from build123d import *

# Parameters (mm, degrees)
F0_W     = 20
F0_H     = 20
F0_W_2   = 9
F0_H_2   = 9
F1_DEPTH = 2
F2_W     = 20
F2_H     = 20
F3_DEPTH = 5.3
F4_R     = 5.25
F5_DEPTH = 10


with BuildPart() as f1:
    # F0 (on Top) → F1 (new body)
    with BuildSketch(Plane.XY):
        Rectangle(F0_W, F0_H)
        Rectangle(F0_W_2, F0_H_2, mode=Mode.SUBTRACT)
    extrude(amount=F1_DEPTH)

    # F2 (on face) → F3 (join)
    with BuildSketch(Plane.XY.offset(2)):
        Rectangle(F2_W, F2_H)
    extrude(amount=F3_DEPTH)

    # F4 (on face) → F5 (cut)
    with BuildSketch(Plane.XY.offset(7.3)):
        Circle(F4_R)
    extrude(amount=-F5_DEPTH, mode=Mode.SUBTRACT)


solid = f1.part
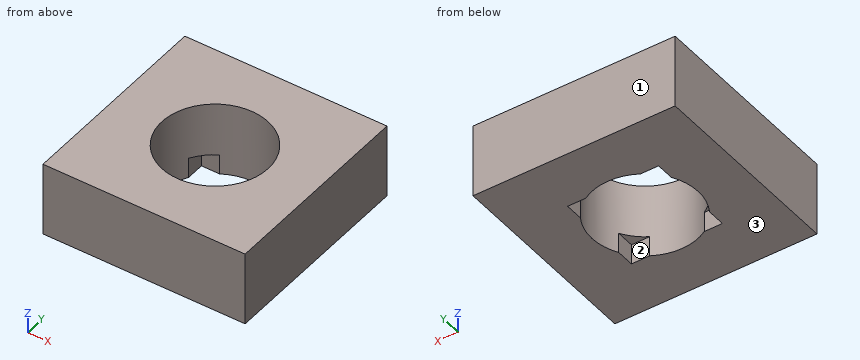
The listing builds one solid part. Answer for the finished solid, in the listing's coordinates (mm). Face numbers are marked on the shaded views. Give positions to 0.01 mm unless a question says otherwise; leave off trailing zeros. Order: outer loops, then holes, each group sorted by start corner. A loop starts at its lowest first (then second) coordinate and runs counter-clockwise, first axis right, second up. Notation, with made-up numbers: (-26.75, 85) - (15.25, 85) arc R14 cw to (15.25, 105) - close; hole circle Ø9 at (40, 6.5). An arc over 180 degrees is marked (long way). Use one line per item in the form item = value.
1) This flat-tipped pin is pushed along its axis until it touches: pin 1 (0.5 mm diameter, centred on x = -3.5, y = 4, fed in from -Z). Where does it stop, or does it pass through?
Verdict:
pin_1 = 2
2) Consider probe 1 along Y at (x, z) = (0, 2.75); probe 2 along Y at (x, z) = (4.5, 4). Determine where each line is inside the solid, lowest interval first. Write a range as [from, to].
Verdict:
probe_1 = [-10, -5.25], [5.25, 10]
probe_2 = [-10, -2.7], [2.7, 10]
3) Find section A-A on y = 0. Determine the outline of the cut face in (x, z), and give its area (4 significant figures).
Verdict:
outline = (-10, 0) - (-5.25, 0) - (-5.25, 7.3) - (-10, 7.3) - close; (5.25, 0) - (10, 0) - (10, 7.3) - (5.25, 7.3) - close
area = 69.35 mm^2
4) The mould has two halves that part along Y. Classify the marked faces 1, 2 and 3: released by +Y, released by -Y, zero draft, split by the parting line, or undercut.
Verdict:
face_1 = released by +Y
face_2 = undercut
face_3 = zero draft
5) Find section C-C on z = 4.25. Determine the outline of the cut face in (x, y), and give its area (3 significant figures).
Verdict:
outline = (-10, -10) - (10, -10) - (10, 10) - (-10, 10) - close; hole circle Ø10.5 at (0, 0)
area = 313 mm^2
